Build history of the part. All positions in model axes, mm. Round coordinates to 2 decimals unless told otherwise and drop trailing zeros. Write each loop counter-clockwise with the first axis right and the second up, starting at its lowest first coordinate (ties: lowest second). Pieces come first, ordered by that corner, then holes.
Item 1: Wall check: probe 1 along X at (y, z) = (-35, 0.6); probe 2 along Y at (x, z) = (24, 0.75) (3 decimals); probe 3 along X at (y, z) = (-14.5, 0.9). Give the ranges that are in metal, low to high.
Item 2: Band-saw the part on B-B, the plane x = 27.75. Write the cut outline in (y, z) (3 decimals).
Item 3: Band-saw the part on C-C, the plane y = -41. Write the cut outline in (x, z), then the cut area to 3 significant figures.
Item 4: Band-saw the part on D-D, the plane x = 35.75. Write the cut outline in (y, z).
Item 5: Band-saw the part on A-A, the plane z = 0.6. Write the cut outline in (x, y) (3 decimals), then the cut area to 3 significant figures.
Item 6: Drop flat-ended pins along their axis: pin 1 Ø0.5 at (x, z) = (40, 0.5) entering from +Y; pin 2 Ø3 at (x, y) = (17.66, -13.29) entering from +Z; pin 3 Ø0.5 at (y, z) = (-41.5, 0.5) entering from +X; pin 4 Ø0.5 at (x, z) = (32.5, 0.5) entering from -Y. Give the stop position or say it passes through.
```python
from build123d import *

# Parameters (mm, degrees)
SKETCH_1_R      = 2.5
EXTRUDE_1_DEPTH = 1


with BuildPart() as part:
    # 스케치1 → 보스-돌출1 (new body)
    with BuildSketch(Plane.XY):
        with BuildLine():
            Line((20.887065526, -4.904042543), (17.65515334, -8.287321674))
            ThreePointArc((17.65515334, -8.287321674), (14.119619434, -9.751787768), (12.65515334, -13.287321674))
            Line((12.65515334, -13.287321674), (12.65515334, -39.724999499))
            Line((12.65515334, -39.724999499), (15.15515334, -39.724999499))
            Line((15.15515334, -39.724999499), (15.15515334, -43.161796007))
            ThreePointArc((15.15515334, -43.161796007), (18.953651475, -43.238083254), (22.731294666, -42.833336733))
            Line((22.731294666, -42.833336733), (22.731294666, -44.249079054))
            Line((22.731294666, -44.249079054), (28.163405743, -44.249079054))
            Line((28.163405743, -44.249079054), (28.163405743, -39.724999499))
            Line((28.163405743, -39.724999499), (25.906714003, -39.724999499))
            Line((25.906714003, -39.724999499), (23.650022264, -39.724999499))
            Line((23.650022264, -39.724999499), (23.650022264, -18.287321674))
            Line((23.650022264, -18.287321674), (37.65515334, -18.287321674))
            ThreePointArc((37.65515334, -18.287321674), (41.190687246, -16.82285558), (42.65515334, -13.287321674))
            Line((42.65515334, -13.287321674), (42.65515334, -9.191405084))
            Line((42.65515334, -9.191405084), (41.15515334, -9.191405084))
            Line((41.15515334, -9.191405084), (41.15515334, -10.336593208))
            Line((41.15515334, -10.336593208), (37.25515334, -10.336593208))
            Line((37.25515334, -10.336593208), (37.25515334, -8.287321674))
            ThreePointArc((37.25515334, -8.287321674), (29.002533556, -6.92744781), (20.887065526, -4.904042543))
        make_face()
        with Locations((17.65515334, -13.287321674)):
            Circle(SKETCH_1_R, mode=Mode.SUBTRACT)
    extrude(amount=EXTRUDE_1_DEPTH)


solid = part.part
```
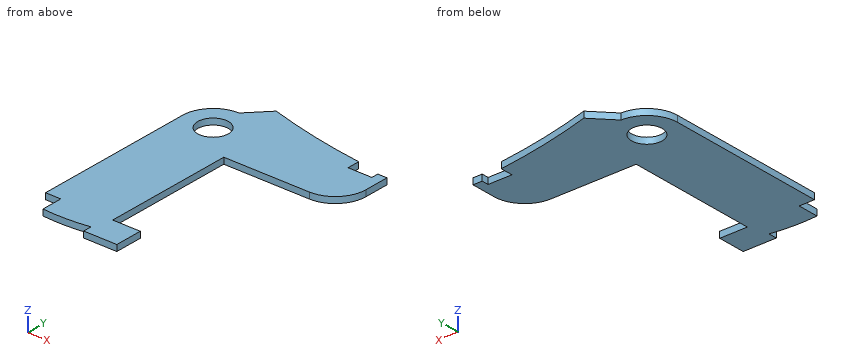
Results:
1. probe 1: x = 12.66 to 23.65
1. probe 2: y = -44.249 to -39.725, -18.287 to -5.763
1. probe 3: x = 12.66 to 15.47, 19.84 to 42.51
2. outline: (-44.249, 0) - (-39.725, 0) - (-39.725, 1) - (-44.249, 1) - close; (-18.287, 0) - (-6.66, 0) - (-6.66, 1) - (-18.287, 1) - close
3. outline: (15.16, 0) - (28.16, 0) - (28.16, 1) - (15.16, 1) - close
3. area: 13.0 mm2
4. outline: (-18.29, 0) - (-8.09, 0) - (-8.09, 1) - (-18.29, 1) - close
5. outline: (12.655, -39.725) - (15.155, -39.725) - (15.155, -43.162) arc R29.979 ccw to (22.731, -42.833) - (22.731, -44.249) - (28.163, -44.249) - (28.163, -39.725) - (23.65, -39.725) - (23.65, -18.287) - (37.655, -18.287) arc R5 ccw to (42.655, -13.287) - (42.655, -9.191) - (41.155, -9.191) - (41.155, -10.337) - (37.255, -10.337) - (37.255, -8.287) arc R103.246 cw to (20.887, -4.904) - (17.655, -8.287) arc R5 ccw to (12.655, -13.287) - close; hole circle Ø5 at (17.655, -13.287)
5. area: 576 mm2
6. pin 1: stops at y = -10.34
6. pin 2: passes through
6. pin 3: stops at x = 28.16
6. pin 4: stops at y = -18.29
